The model under review builds one solid part; all positions refer to its coordinate system, in mm. Face numbers are marked on the shaded views. A direction names the side the tool comes from. Coordinates: 2 decimals unless noted, no trailing zeros. Order: outer loops, then holes, each group sorted by start corner. A loop starts at its lowest first (then second) coordinate and runs counter-clockwise, first axis right, second up. Notation, with made-up numbers: M 58.5,10.25 L 84.5,10.25 A22 ccw 84.5,16.25 Z; hole C 36.25,12 d1. An arc over 180 degrees is marked long. Answer as CSV lines item,"result". Start each with the question number.
Q1. For P1, Ø4, axis at y = 4.5, z = -8.5, coming from the -X side; P2, Ø4, axis at y = 1, z = -20, coming from the +X side; P3, Ø3.5, axis at y = 1.5, z = 1, coming from the -X side, all flat-tipped, find the tip position at first contact; note any pin that passes through.
Q2. The part is to be moulded in two halves that separate along Z. For the marked faces 4, 5, 6 and 7, say which applies: +Z half, -Z half, draft (parallel to the pull), parting line (faces both ways), or undercut.
Q3. Consider section B-B on z = -11.5. Write out the cut boundary in (x, y).
Q4. Consider section D-D on x = -4. Write out the cut boundary in (y, z), and give its area (3 significant figures).
Q5. Consider section A-A on x = 12. Write out the cut boundary in (y, z), and give its area (3 significant figures).
Q6. Machinability: for the marked faces 1, 2 and 3, which of the approach directions +Z, -Z, +X, -X, +Y, -Y give a long, thin tool a straight path to every point of the face, cutting with its end or side? Answer none if there is none.
Q7. Wall thickness on L1, parallel to Y at x = 12, z = -23.9; L2, parallel to Z at x = 10, y = 5.5; L3, parallel to Y at x = 12, z = 2.5: over which ranges is each line inside the solid? List them lowest first. Write a range as [from, to].
Q8. Consider section C-C on y = 0. State how many separate pieces and enclosed holes the cut face has, and give its area (3 significant figures).
from build123d import *

# Parameters (mm, degrees)
F1_DEPTH       = 15
F2_R           = 5
F3_R           = 10
F5_D           = 4.2
F5_CSINK_D     = 8
F5_CSINK_ANGLE = 90
F6_R           = 5
F7_DEPTH       = 5
F8_T1_DEPTH    = 47.7203429425
F9_R           = 2
F10_SIZE       = 5


# Not quite as in the source:
# - a fillet or chamfer that OpenCascade refuses, or shapes differently, is made with other operations: its cross-section is extruded or revolved along the edge and cut away or added


with BuildPart() as f1:
    # F0 (on Front) → F1 (new body, symmetric)
    with BuildSketch(Plane.XZ):
        Polygon((0, 3), (0, 0), (30, 0), (30, -20), (-15, -20), (-23.6602540378, -15), (-25.0838401426, -16.1945305755), (-20, -25), (35, -25), (35, 3), align=None)
    extrude(amount=F1_DEPTH, both=True)

    # F2
    f2_edges = [f1.edges().sort_by_distance(p)[0] for p in [
        (30, 0, 0),
        (30, 0, -20),
        (-15, 0, -20),
    ]]
    fillet(f2_edges, radius=F2_R)

    # F3
    f3_edges = [f1.edges().sort_by_distance(p)[0] for p in [
        (35, 0, 3),
        (35, 0, -25),
        (-20, 0, -25),
    ]]
    fillet(f3_edges, radius=F3_R)

    # F5 (through all)
    with Locations(Plane(origin=(0, 0, 0), x_dir=(1, 0, 0), z_dir=(0, 0, -1))):
        with Locations((12, 0)):
            CounterSinkHole(F5_D / 2, F5_CSINK_D / 2, counter_sink_angle=F5_CSINK_ANGLE)

    # F6 (on face) → F7 (cut, through all)
    with BuildSketch(Plane(origin=(0, 0, -25), x_dir=(1, 0, 0), z_dir=(0, 0, -1))):
        with Locations((12, 0)):
            Circle(F6_R)
    extrude(amount=-F7_DEPTH, mode=Mode.SUBTRACT)

    # F8: fillet of radius 5 on 1 edges, made by hand

    # F8_s2 → F8_t1 (cut)
    with BuildSketch(Plane.XZ.offset(-23.8601714713)):
        with BuildLine():
            ThreePointArc((-23.3118058484, -19.2637840059), (-23.9650654758, -17.171040108), (-23.6602540378, -15))
            Line((-23.6602540378, -15), (-25.0838401426, -16.1945305755))
            Line((-25.0838401426, -16.1945305755), (-23.3118058484, -19.2637840059))
        make_face()
    extrude(amount=F8_T1_DEPTH, mode=Mode.SUBTRACT)

    # F9
    f9_edges = [f1.edges().sort_by_distance(p)[0] for p in [
        (-23.660254, 0, -15),
    ]]
    fillet(f9_edges, radius=F9_R)

    # F10
    f10_edges = [f1.edges().sort_by_distance(p)[0] for p in [
        (0, 15, 1.5),
        (0, -15, 1.5),
    ]]
    chamfer(f10_edges, length=F10_SIZE)


solid = f1.part
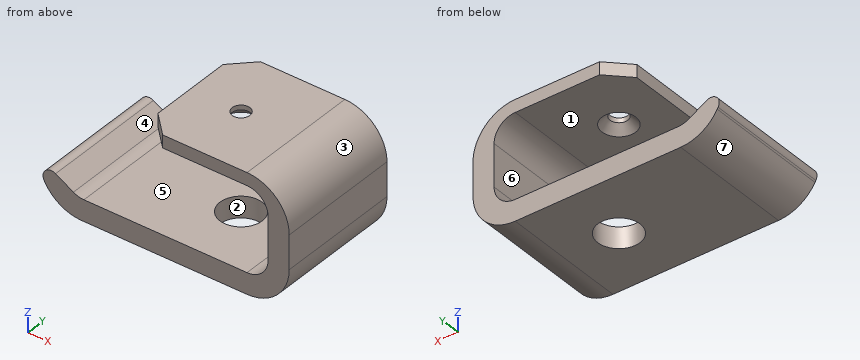
Evaluation:
1,P1,"stops at x = 30"
1,P2,"stops at x = 34.54"
1,P3,"stops at x = 0"
2,face 4,"+Z half"
2,face 5,"undercut"
2,face 6,"undercut"
2,face 7,"-Z half"
3,outline,"M 30,-15 L 35,-15 L 35,15 L 30,15 Z"
4,outline,"M -15,-25 L 15,-25 L 15,-20 L -15,-20 Z"
4,area,"150 mm²"
5,outline,"M -15,-25 L -5,-25 L -5,-20 L -15,-20 Z; M -15,0 L -4,0 L -2.1,1.9 L -2.1,3 L -15,3 Z; M 2.1,1.9 L 4,0 L 15,0 L 15,3 L 2.1,3 Z; M 5,-25 L 15,-25 L 15,-20 L 5,-20 Z"
5,area,"174 mm²"
6,face 1,"-X, +Y, -Y"
6,face 2,"-Z"
6,face 3,"+Z, +X, +Y, -Y"
7,L1,"y = [-15, -5], [5, 15]"
7,L2,"z = [-25, -20], [0, 3]"
7,L3,"y = [-15, -2.1], [2.1, 15]"
8,separate pieces,"3"
8,enclosed holes,"0"
8,area,"401 mm²"
